Build history of the part. All positions in model axes, mm. Face numbers are marked on the shaded views. Coordinates: 2 decimals unless noted, no trailing zeros. Order: outer loops, then holes, each group sorted by start corner. A loop starts at its lowest first (then second) coordinate and runs counter-clockwise, first axis right, second up. Notation, with made-up numbers: (80.5, 16.25) - (128.5, 16.25) arc R12 ccw to (128.5, 35.25) - close; hole circle Ø2 at (19.5, -40). An arc over 180 degrees is marked (long way). Return JSON: item names as keys, results as strings.
from build123d import *

# Parameters (mm, degrees)
BOSS_EXTRUDE1_DEPTH = 5
SKETCH3_W           = 80
SKETCH3_H           = 5
BOSS_EXTRUDE2_DEPTH = 5
SKETCH6_W           = 80
SKETCH6_H           = 5
SKETCH6_W_2         = 74.5
SKETCH6_H_2         = 2.1
CUT_EXTRUDE2_DEPTH  = 2.5
FILLET1_R           = 10
SKETCH7_R           = 2.9
CUT_EXTRUDE3_DEPTH  = 5
SKETCH8_R           = 1.7
CUT_EXTRUDE4_DEPTH  = 5
CIRPATTERN1_COUNT   = 4
SKETCH9_R           = 10.25
CUT_EXTRUDE5_DEPTH  = 2.5


with BuildPart() as part:
    # Sketch2 → Boss-Extrude1 (new body)
    with BuildSketch(Plane(origin=(0, 0, 0), x_dir=(1, 0, 0), z_dir=(0, 1, 0))):
        with BuildLine():
            Line((-40, 0), (40, 0))
            Line((40, 0), (13.582225242, -56.365780194))
            ThreePointArc((13.582225242, -56.365780194), (0, -65), (-13.582225242, -56.365780194))
            Line((-13.582225242, -56.365780194), (-40, 0))
        make_face()
    extrude(amount=BOSS_EXTRUDE1_DEPTH)

    # Sketch3 → Boss-Extrude2 (add)
    with BuildSketch(Plane(origin=(0, 0, 0), x_dir=(-1, 0, 0), z_dir=(0, 0, -1))):
        with Locations((0, 2.5)):
            Rectangle(SKETCH3_W, SKETCH3_H)
    extrude(amount=BOSS_EXTRUDE2_DEPTH)

    # Sketch6 → Cut-Extrude2 (cut)
    with BuildSketch(Plane(origin=(0, 0, -5), x_dir=(-1, 0, 0), z_dir=(0, 0, -1))):
        with Locations((0, 2.5)):
            Rectangle(SKETCH6_W, SKETCH6_H)
        with Locations((0, 2.5)):
            Rectangle(SKETCH6_W_2, SKETCH6_H_2, mode=Mode.SUBTRACT)
    extrude(amount=-CUT_EXTRUDE2_DEPTH, mode=Mode.SUBTRACT)

    # Fillet1
    fillet1_edges = [part.edges().sort_by_distance(p)[0] for p in [
        (-40, 2.5, 0),
        (40, 2.5, 0),
    ]]
    fillet(fillet1_edges, radius=FILLET1_R)

    # Sketch7 → Cut-Extrude3 (cut)
    with BuildSketch(Plane(origin=(0, 0, 0), x_dir=(-1, 0, 0), z_dir=(0, -1, 0))):
        with Locations(Location((0, -50, 0), (0, 0, 90))):
            Circle(SKETCH7_R)
    extrude(amount=-CUT_EXTRUDE3_DEPTH, mode=Mode.SUBTRACT)

    # Sketch8 → Cut-Extrude4 (cut)
    with BuildSketch(Plane(origin=(0, 5, 0), x_dir=(1, 0, 0), z_dir=(0, 1, 0))):
        with Locations(Location((0, -57, 0), (0, 0, 270))):
            Circle(SKETCH8_R)
    cut_extrude4 = extrude(amount=-CUT_EXTRUDE4_DEPTH, mode=Mode.SUBTRACT)

    # CirPattern1: Cut-Extrude4 ×4 about axis
    cirpattern1_axis = Axis((0, 0, 50), (0, 1, 0))
    for i in range(1, CIRPATTERN1_COUNT):
        add(cut_extrude4.rotate(cirpattern1_axis, i * 360 / CIRPATTERN1_COUNT), mode=Mode.SUBTRACT)

    # Sketch9 → Cut-Extrude5 (cut)
    with BuildSketch(Plane(origin=(0, 5, 0), x_dir=(1, 0, 0), z_dir=(0, 1, 0))):
        with Locations(Location((0, -50, 0), (0, 0, 270))):
            Circle(SKETCH9_R)
    extrude(amount=-CUT_EXTRUDE5_DEPTH, mode=Mode.SUBTRACT)


solid = part.part
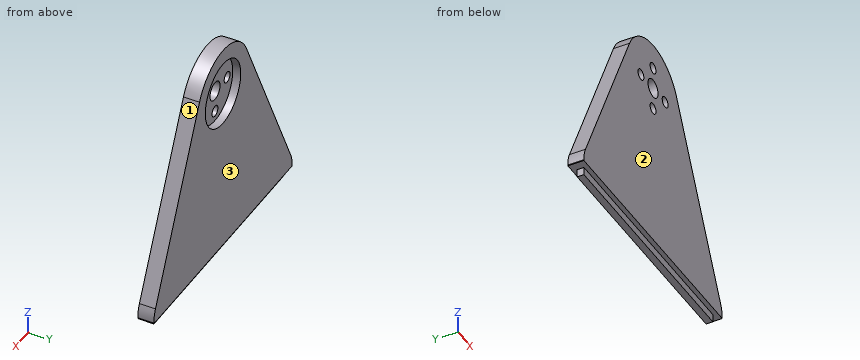
1. Mould opens along Y. For the marked faces 1, 2 and 3 say: pulls with the +Y half, pulls with the -Y half, needs draft (parallel to the pull), parting line crosses it, or undercut.
Check values:
{"face 1": "needs draft", "face 2": "pulls with the -Y half", "face 3": "pulls with the +Y half"}
2. Drop flat-ended pins along their axis: pin 1 (1.2 mm diameter, centred on x = -10.5, z = -4, fed in from -Y); pin 2 (1.7 mm diameter, centred on y = 2.5, z = -3.5, fed in from -X); pin 3 (0.8 mm diameter, centred on x = 9.5, z = -4, fed in from +Y). Give the stop position or say it passes through.
Check values:
{"pin 1": "y = 1.45", "pin 2": "x = -37.25", "pin 3": "y = 3.55"}
3. Cut at A-A on x = 0. Give the cut face in (y, z), plus the area to 3 significant figures.
Check values:
{"outline": "(0, -2.5) - (1.45, -2.5) - (1.45, -5) - (3.55, -5) - (3.55, -2.5) - (5, -2.5) - (5, 39.75) - (2.5, 39.75) - (2.5, 41.3) - (0, 41.3) - close; (0, 44.7) - (2.5, 44.7) - (2.5, 47.1) - (0, 47.1) - close; (0, 52.9) - (2.5, 52.9) - (2.5, 55.3) - (0, 55.3) - close; (0, 58.7) - (2.5, 58.7) - (2.5, 60.25) - (5, 60.25) - (5, 65) - (0, 65) - close", "area": "260 mm²"}
4. Cut at D-D on x = 28.5. Give the cut face in (y, z), plus the area to 3 significant figures.
Check values:
{"outline": "(0, -2.5) - (1.45, -2.5) - (1.45, -5) - (3.55, -5) - (3.55, -2.5) - (5, -2.5) - (5, 24.54) - (0, 24.54) - close", "area": "140 mm²"}
5. Probe L1, parallel to X at y = 0.9, z = 49; L2, parallel to Z at x = 7, y = 1.6; L3, parallel to Z at x = 6.5, y = 4.6. List the from-to ranges inside material, lowest first.
Check values:
{"L1": "-17.03 to -8.37, -5.63 to -2.72, 2.72 to 5.63, 8.37 to 17.03", "L2": "-5 to 48.3, 51.7 to 63.27", "L3": "-2.5 to 42.07, 57.93 to 63.52"}
6. Cut at B-B on z = 50. Give the cut face in (x, y), plus the area to 3 significant figures.
Check values:
{"outline": "(-16.57, 0) - (-8.7, 0) - (-8.7, 2.5) - (-10.25, 2.5) - (-10.25, 5) - (-16.57, 5) - close; (-5.3, 0) - (-2.9, 0) - (-2.9, 2.5) - (-5.3, 2.5) - close; (2.9, 0) - (5.3, 0) - (5.3, 2.5) - (2.9, 2.5) - close; (8.7, 0) - (16.57, 0) - (16.57, 5) - (10.25, 5) - (10.25, 2.5) - (8.7, 2.5) - close", "area": "82.9 mm²"}
7. Cut at C-C on z = 43. Give the cut face in (x, y).
Check values:
{"outline": "(-19.85, 0) - (-1.7, 0) - (-1.7, 2.5) - (-7.49, 2.5) - (-7.49, 5) - (-19.85, 5) - close; (1.7, 0) - (19.85, 0) - (19.85, 5) - (7.49, 5) - (7.49, 2.5) - (1.7, 2.5) - close"}
